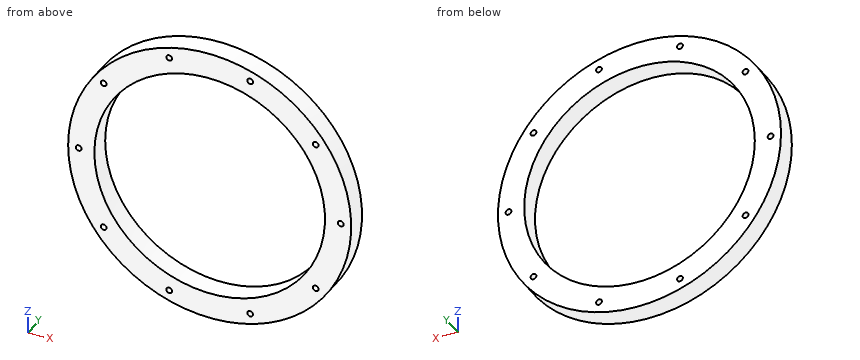
Autodesk Inventor part; units mm, degrees
ref_plane "YZ Plane" through (0, 0, 0) normal (1, 0, 0) x (0, 1, 0)
ref_plane "XZ Plane" through (0, 0, 0) normal (0, 1, 0) x (-1, 0, 0)
ref_plane "XY Plane" through (0, 0, 0) normal (0, 0, 1) x (1, 0, 0)
sketch "Sketch1" plane through (0, 0, 0) normal (0, 1, 0) x (-1, 0, 0)
  circle A0 centre (0, 0) radius 135
  circle A1 centre (0, 0) radius 110
  dimension "d0" = 270
  dimension "d1" = 220
extrude "Extrusion1" add sketch "Sketch1" along normal mid plane 20
sketch "Sketch3" plane through (0, 10, 0) normal (0, 1, 0) x (1, 0, 0)
  circle A0 centre (0, 0) radius 125
  circle A1 centre (125, 0) radius 2.5
  circle A2 centre (101.1271, 73.4732) radius 2.5
  circle A3 centre (38.6271, 118.8821) radius 2.5
  circle A4 centre (-38.6271, 118.8821) radius 2.5
  circle A5 centre (-101.1271, 73.4732) radius 2.5
  circle A6 centre (-125, 0) radius 2.5
  circle A7 centre (-101.1271, -73.4732) radius 2.5
  circle A8 centre (-38.6271, -118.8821) radius 2.5
  circle A9 centre (38.6271, -118.8821) radius 2.5
  circle A10 centre (101.1271, -73.4732) radius 2.5
  dimension "d7" = 250
  dimension "d8" = 5
  dimension "d11" = 360
hole "Hole1" at (125, 10, 0) at (101.1271, 10, 73.4732) at (38.6271, 10, 118.8821) at (-38.6271, 10, 118.8821) at (-101.1271, 10, 73.4732) at (-125, 10, 0) at (-101.1271, 10, -73.4732) at (-38.6271, 10, -118.8821) at (38.6271, 10, -118.8821) at (101.1271, 10, -73.4732) direction (0, -1, 0) diameter 5.5 end through all
properties part number "Cylinder Spacer (x3)"
Geometry: final body of the model. Coordinates: model frame, mm. Round coordinates to 2 decimals unless told otherwise and drop trailing zeros. Write each loop counter-clockwise with the first axis right and the second up, starting at its lowest first coordinate (ties: lowest second). Pieces come first, ordered by that corner, then holes. Notation, with made-up numbers: (-4.75, 50.25) -> (33.25, 50.25) arc R26 ccw to (33.25, 64.25) -> close; hole circle Ø4 at (85, 8.25). An arc over 180 degrees is marked (long way). Return JSON: item names as keys, results as strings.
Q1. Section C-C on y = 3.25. Give the number of separate pieces and of enclosed holes in the cut face, and give its area (3 significant figures).
From the geometry:
{"separate pieces": "1", "enclosed holes": "11", "area": "19,000 mm2"}
Q2. Ray query, line 1 (X direction, y = 0.25, z = -119.5); line 2 (Z direction, x = 40, y = 4.5); line 3 (Z direction, x = 36.5, y = -3.5). Return the intervals inside material, ascending.
From the geometry:
{"line 1": "-62.81 to -41.31, -35.95 to 35.95, 41.31 to 62.81", "line 2": "-128.94 to -121.26, -116.5 to -102.47, 102.47 to 116.5, 121.26 to 128.94", "line 3": "-129.97 to -120.63, -117.14 to -103.77, 103.77 to 117.14, 120.63 to 129.97"}
Q3. Section B-B on z = -46.5. Return the cut outline in (x, y), and give its area (3 significant figures).
From the geometry:
{"outline": "(-126.74, -10) -> (-99.69, -10) -> (-99.69, 10) -> (-126.74, 10) -> close; (99.69, -10) -> (126.74, -10) -> (126.74, 10) -> (99.69, 10) -> close", "area": "1,080 mm2"}
Q4. First-contact query: pin 1 Ø5 at (x, y) = (-8.5, 4.5) entering from +Z; pin 2 Ø2 at (y, z) = (-7.5, 89.5) entering from -X; pin 3 Ø8 at (y, z) = (-4, -96.5) entering from -X. Flat tips, straight axial feed; report the tip coordinate or a pass-through.
From the geometry:
{"pin 1": "z = 134.87", "pin 2": "x = -101.94", "pin 3": "x = -98.33"}
Q5. Section A-A on x = 0. Return the cut outline in (y, z).
From the geometry:
{"outline": "(-10, -135) -> (10, -135) -> (10, -110) -> (-10, -110) -> close; (-10, 110) -> (10, 110) -> (10, 135) -> (-10, 135) -> close"}
